Answer from the drawing. Dimensions are ordinates in mm from the lowest x, y and z of the part. A direction names the side the tool comes from. Round coordinates to 2 decimals unless told otherwise and drop trailing zeros. Loops run counter-clockwise (first coordinate to the right, second up) from the corner with the lowest first, then second, coordinate; pieces in that order, holes last.
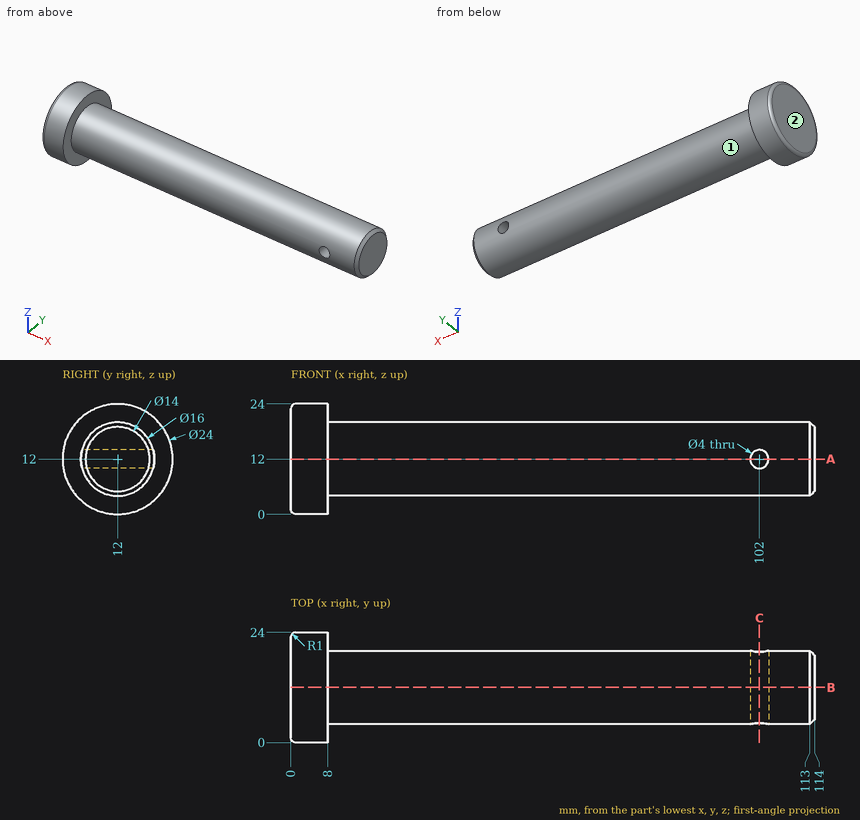
1. Which of the six approach directions +Z, -Z, +X, -X, +Y, -Y give full straight-line access (tool end or side, diameter ignored) to the marked faces 1 and 2?
Answer key:
face 1: +X
face 2: +Z, -Z, -X, +Y, -Y
2. Find section A-A (z = 12). Write down the section's boundary in (x, y).
Answer key:
outline: (0, 1) arc R1 ccw to (1, 0) - (8, 0) - (8, 4) - (100, 4) - (100, 20) - (8, 20) - (8, 24) - (1, 24) arc R1 ccw to (0, 23) - close; (104, 4) - (113, 4) - (114, 5) - (114, 19) - (113, 20) - (104, 20) - close
3. Find section C-C (x = 102). Write down the section's boundary in (y, z).
Answer key:
outline: (4.25, 10) arc R8 ccw to (19.75, 10) - close; (4.25, 14) - (19.75, 14) arc R8 ccw to start
4. Given pin 1 (1 mm diameter, centred on x = 23, z = 19, fed in from -Y); pin 2 (12 mm diameter, centred on x = 39, z = 18.5, fed in from +Y); pin 3 (3 mm diameter, centred on x = 44.5, y = 7, fed in from -Z), each flat-ended and moving along its own axis, determine where each tip first touches the part or whether it passes through.
Answer key:
pin 1: stops at y = 7.34
pin 2: stops at y = 19.98
pin 3: stops at z = 4.81
5. Find section B-B (y = 12). Write down the section's boundary in (x, z), then the cut area to 3 significant figures.
Answer key:
outline: (0, 1) arc R1 ccw to (1, 0) - (8, 0) - (8, 4) - (113, 4) - (114, 5) - (114, 19) - (113, 20) - (8, 20) - (8, 24) - (1, 24) arc R1 ccw to (0, 23) - close; hole circle Ø4 at (102, 12)
area: 1,870 mm2
6. Consider probe 1 along X at (y, z) = (13.5, 12); probe 2 along X at (y, z) = (11, 20); probe 3 along Z at (x, y) = (46, 12.5). Determine where each line is inside the solid, lowest interval first.
Answer key:
probe 1: x = 0 to 100, 104 to 114
probe 2: x = 0 to 8
probe 3: z = 4.02 to 19.98
